```python
from build123d import *

# Parameters (mm, degrees)
SKETCH1_R           = 5
BOSS_EXTRUDE1_DEPTH = 5


with BuildPart() as part:
    # Sketch1 → Boss-Extrude1 (new, symmetric)
    with BuildSketch(Plane.XY):
        with BuildLine():
            Line((320, 39), (300, 39))
            Line((300, 39), (300, 9))
            Line((300, 9), (320, 9))
            ThreePointArc((320, 9), (335, 24), (320, 39))
        make_face()
        with Locations((320, 24)):
            Circle(SKETCH1_R, mode=Mode.SUBTRACT)
    extrude(amount=BOSS_EXTRUDE1_DEPTH, both=True)

    # Sketch4 → Revolve2 (revolve)
    with BuildSketch(Plane.XY, mode=Mode.PRIVATE) as revolve2_sk:
        Polygon((300, 39), (300, 48.198468166), (158.764392762, 48.198468166), (158.764392762, 39), (289.025351805, 39), (289.025351805, 24), (300, 24), align=None)
    revolve(revolve2_sk.sketch.rotate(Axis((289.025351805, 24, 0), (1, 0, 0)), 90), axis=Axis((289.025351805, 24, 0), (1, 0, 0)))


solid = part.part
```
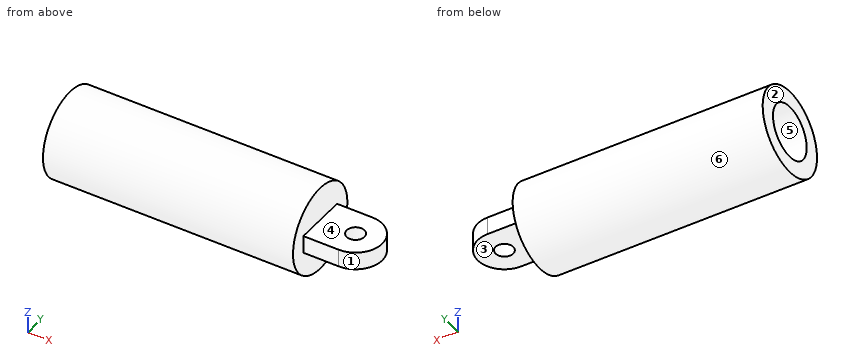
For this review, take the finished solid that the model builds, in its own axes (mm). Face numbers are marked on the shaded views. A direction names the side the tool comes from. Round coordinates to 2 decimals unless told otherwise and drop trailing zeros. Order: outer loops, then holes, each group sorted by start corner. A loop starts at its lowest first (then second) coordinate and runs counter-clockwise, first axis right, second up. Notation, with made-up numbers: (-29, -21) -> (9, -21) arc R27 ccw to (9, 17) -> close; hole circle Ø5 at (-22.5, -39.5). An arc over 180 degrees is marked (long way). Use a Markdown table: item, result.
Item 1: Take a section at A-A (y = 24). State the section outline as (x, z) points.
Resolved:
| item | result |
|---|---|
| outline | (158.76, -24.2) -> (300, -24.2) -> (300, -5) -> (315, -5) -> (315, 5) -> (300, 5) -> (300, 24.2) -> (158.76, 24.2) -> (158.76, 15) -> (289.03, 15) -> (289.03, -15) -> (158.76, -15) -> close; (325, -5) -> (335, -5) -> (335, 5) -> (325, 5) -> close |
Item 2: For pin 1 (1.5 mm diameter, centred on y = 32, z = 9.5, fed in from -X); pin 2 (1 mm diameter, centred on x = 187, z = -16.5, fed in from -Y); pin 3 (6 mm diameter, centred on y = 34, z = 15, fed in from +X); pin 4 (8 mm diameter, centred on x = 320, y = 24, fed in from +Z), all flat-tipped, find the tip position at first contact; note any pin that passes through.
Resolved:
| item | result |
|---|---|
| pin 1 | stops at x = 289.03 |
| pin 2 | stops at y = 5.85 |
| pin 3 | stops at x = 300 |
| pin 4 | passes through |
Item 3: Machinability: for the marked faces 4, 5 and 6, which of the approach directions +Z, -Z, +X, -X, +Y, -Y give a long, thin tool a straight path to every point of the face, cutting with its end or side? Answer none if there is none.
Resolved:
| item | result |
|---|---|
| face 4 | +Z, +X, +Y, -Y |
| face 5 | -X |
| face 6 | +X, -X |
Item 4: Draft analysis for pull direction X (two halves, no side actions). For the marked faces 1, 2 and 3, state which applies: +X half, -X half, draft (parallel to the pull), parting line (faces both ways), or undercut.
Resolved:
| item | result |
|---|---|
| face 1 | +X half |
| face 2 | -X half |
| face 3 | draft |
Item 5: Take a section at C-C (x = 193). State the section outline as (y, z) points.
Resolved:
| item | result |
|---|---|
| outline | circle Ø48.4 at (24, 0); hole circle Ø30 at (24, 0) |
Item 6: Take a section at D-D (y = 36). State the section outline as (x, z) points.
Resolved:
| item | result |
|---|---|
| outline | (158.76, -21.01) -> (300, -21.01) -> (300, -5) -> (329, -5) -> (329, 5) -> (300, 5) -> (300, 21.01) -> (158.76, 21.01) -> (158.76, 9) -> (289.03, 9) -> (289.03, -9) -> (158.76, -9) -> close |
Item 7: Take a section at B-B (z = 0). State the section outline as (x, y) points, plus the area to 3 significant figures.
Resolved:
| item | result |
|---|---|
| outline | (158.76, -0.2) -> (300, -0.2) -> (300, 9) -> (320, 9) arc R15 ccw to (320, 39) -> (300, 39) -> (300, 48.2) -> (158.76, 48.2) -> (158.76, 39) -> (289.03, 39) -> (289.03, 9) -> (158.76, 9) -> close; hole circle Ø10 at (320, 24) |
| area | 3,800 mm² |
Item 8: For line 1 along Y through (x, z) = (320, 1); line 2 along Z through (x, y) = (187.5, 25); line 3 along Y through (x, z) = (262, -1), list the stretches that pass through material, from the lowest coordinate up. Write a range as [from, to].
Resolved:
| item | result |
|---|---|
| line 1 | y = [9, 19], [29, 39] |
| line 2 | z = [-24.18, -14.97], [14.97, 24.18] |
| line 3 | y = [-0.18, 9.03], [38.97, 48.18] |
